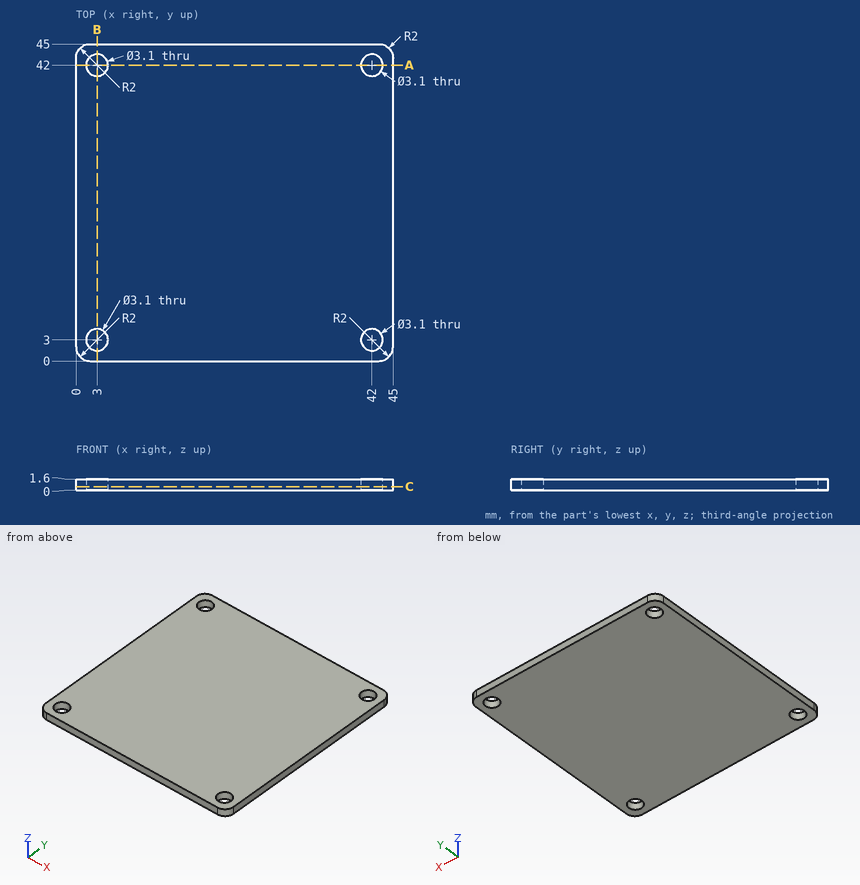
Check sheet for the drawn part. Datum: minimum x, y, z corner. Units: mm. Round coordinates to 2 decimals unless told otherwise and drop trailing zeros. Loops run counter-clockwise (first coordinate to the right, second up) from the corner with the lowest first, then second, coordinate; pieces in that order, holes last. Notation, with made-up numbers: (89, -25.5) - (100, -25.5) arc R26 cw to (100, -11.5) - close; hole circle Ø11 at (-13, -4.75). An arc over 180 degrees is marked (long way). Write item = value, one per line. Start each with the question number.
1. Section check C-C on z = 0.5. Enter the section's corners in (x, y).
2. Thickness scan on line 1 (Y direction, x = 42, z = 0.65). Record the ranges inside material, lowest first.
3. Depth check by flat-ended pin: pin 1 (3 mm diameter, centred on x = 3, y = 42, fed in from +Z). Enter the tip coordinate at first touch or a pass-through.
4. Section check A-A on y = 42. Enter the section's corners in (x, z), then the cut area to 3 significant figures.
Working result:
q1.outline = (0, 2) arc R2 ccw to (2, 0) - (43, 0) arc R2 ccw to (45, 2) - (45, 43) arc R2 ccw to (43, 45) - (2, 45) arc R2 ccw to (0, 43) - close; hole circle Ø3.1 at (3, 3); hole circle Ø3.1 at (3, 42); hole circle Ø3.1 at (42, 3); hole circle Ø3.1 at (42, 42)
q2.line_1 = 0 to 1.45, 4.55 to 40.45, 43.55 to 45
q3.pin_1 = through
q4.outline = (0, 0) - (1.45, 0) - (1.45, 1.6) - (0, 1.6) - close; (4.55, 0) - (40.45, 0) - (40.45, 1.6) - (4.55, 1.6) - close; (43.55, 0) - (45, 0) - (45, 1.6) - (43.55, 1.6) - close
q4.area = 62.1 mm^2
